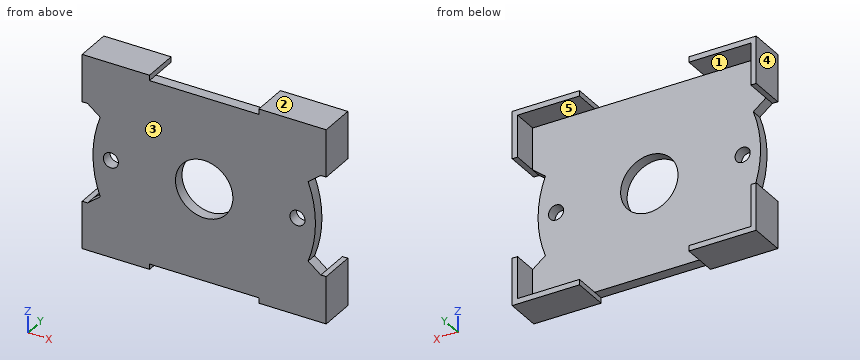
```python
from build123d import *

# Parameters (mm, degrees)
BOSS_EXTRUDE1_DEPTH   = 10
BOSS_EXTRUDE1_2_DEPTH = 10
BOSS_EXTRUDE1_3_DEPTH = 10
BOSS_EXTRUDE1_4_DEPTH = 10
SKETCH1_9_R           = 2.1
SKETCH1_9_R_2         = 22.5
SKETCH1_9_R_3         = 8
BOSS_EXTRUDE2_DEPTH   = 3


with BuildPart() as part:
    # Sketch1 → Boss-Extrude1 (new body)
    with BuildSketch(Plane(origin=(0, 0, 0), x_dir=(1, 0, 0), z_dir=(0, 1, 0))):
        Polygon((-15.231546212, -27), (-15.231546212, -25.5), (-17.628102564, -25.5), (-32.5, -25.5), (-32.5, -13.831280473), (-34, -13.831280473), (-34, -27), align=None)
    extrude(amount=BOSS_EXTRUDE1_DEPTH)



with BuildPart() as body_2:
    # Sketch1 → Boss-Extrude1 2 (new body)
    with BuildSketch(Plane(origin=(0, 0, 0), x_dir=(1, 0, 0), z_dir=(0, 1, 0))):
        Polygon((32.5, -13.831280473), (32.5, -25.5), (17.628102564, -25.5), (15.231546212, -25.5), (15.231546212, -27), (34, -27), (34, -13.831280473), align=None)
    extrude(amount=BOSS_EXTRUDE1_2_DEPTH)


with BuildPart() as body_3:
    # Sketch1 → Boss-Extrude1 3 (new body)
    with BuildSketch(Plane(origin=(0, 0, 0), x_dir=(1, 0, 0), z_dir=(0, 1, 0))):
        Polygon((32.5, 25.5), (32.5, 13.831280473), (34, 13.831280473), (34, 27), (15.231546212, 27), (15.231546212, 25.5), (17.628102564, 25.5), align=None)
    extrude(amount=BOSS_EXTRUDE1_3_DEPTH)


with BuildPart() as body_4:
    # Sketch1 → Boss-Extrude1 4 (new body)
    with BuildSketch(Plane(origin=(0, 0, 0), x_dir=(1, 0, 0), z_dir=(0, 1, 0))):
        Polygon((-17.628102564, 25.5), (-15.231546212, 25.5), (-15.231546212, 27), (-34, 27), (-34, 13.831280473), (-32.5, 13.831280473), (-32.5, 25.5), align=None)
    extrude(amount=BOSS_EXTRUDE1_4_DEPTH)


with BuildPart() as part_1:
    add(part.part)

    add(body_2.part)  # Boss-Extrude2 merges body 2

    add(body_3.part)  # Boss-Extrude2 merges body 3

    add(body_4.part)  # Boss-Extrude2 merges body 4
    # Sketch1_9 → Boss-Extrude2 (add)
    # profile 1 of 15: a face of its own
    with BuildSketch(Plane(origin=(0, 0, 0), x_dir=(1, 0, 0), z_dir=(0, 1, 0))):
        with BuildLine():
            Line((-32.5, 25.5), (-32.5, 13.831280473))
            Line((-32.5, 13.831280473), (-28.961769494, 11.055130384))
            ThreePointArc((-28.961769494, 11.055130384), (-24.388882901, 19.135892737), (-17.628102564, 25.5))
            Line((-17.628102564, 25.5), (-32.5, 25.5))
        make_face()
    # profile 2 of 15: a face of its own
    with BuildSketch(Plane(origin=(0, 0, 0), x_dir=(1, 0, 0), z_dir=(0, 1, 0))):
        with BuildLine():
            Line((-28.961769494, 11.055130384), (-21.828002387, 5.457866962))
            ThreePointArc((-21.828002387, 5.457866962), (-17.701608557, 13.888954406), (-10.494335458, 19.902736578))
            Line((-10.494335458, 19.902736578), (-17.628102564, 25.5))
            ThreePointArc((-17.628102564, 25.5), (-24.388882901, 19.135892737), (-28.961769494, 11.055130384))
        make_face()
    # profile 3 of 15: a face of its own
    with BuildSketch(Plane(origin=(0, 0, 0), x_dir=(1, 0, 0), z_dir=(0, 1, 0))):
        with BuildLine():
            Line((10.494335458, 19.902736578), (17.628102564, 25.5))
            Line((17.628102564, 25.5), (15.231546212, 25.5))
            Line((15.231546212, 25.5), (-15.231546212, 25.5))
            Line((-15.231546212, 25.5), (-17.628102564, 25.5))
            Line((-17.628102564, 25.5), (-10.494335458, 19.902736578))
            ThreePointArc((-10.494335458, 19.902736578), (0, 22.5), (10.494335458, 19.902736578))
        make_face()
    # profile 4 of 15: a face of its own
    with BuildSketch(Plane(origin=(0, 0, 0), x_dir=(1, 0, 0), z_dir=(0, 1, 0))):
        with BuildLine():
            Line((21.828002387, 5.457866962), (28.961769494, 11.055130384))
            ThreePointArc((28.961769494, 11.055130384), (24.388882901, 19.135892737), (17.628102564, 25.5))
            Line((17.628102564, 25.5), (10.494335458, 19.902736578))
            ThreePointArc((10.494335458, 19.902736578), (17.701608557, 13.888954406), (21.828002387, 5.457866962))
        make_face()
    # profile 5 of 15: a face of its own
    with BuildSketch(Plane(origin=(0, 0, 0), x_dir=(1, 0, 0), z_dir=(0, 1, 0))):
        with BuildLine():
            Line((28.961769494, 11.055130384), (32.5, 13.831280473))
            Line((32.5, 13.831280473), (32.5, 25.5))
            Line((32.5, 25.5), (17.628102564, 25.5))
            ThreePointArc((17.628102564, 25.5), (24.388882901, 19.135892737), (28.961769494, 11.055130384))
        make_face()
    # profile 6 of 15: a face of its own
    with BuildSketch(Plane(origin=(0, 0, 0), x_dir=(1, 0, 0), z_dir=(0, 1, 0))):
        with BuildLine():
            Line((21.828002387, -5.457866962), (28.961769494, -11.055130384))
            ThreePointArc((28.961769494, -11.055130384), (31, 0), (28.961769494, 11.055130384))
            Line((28.961769494, 11.055130384), (21.828002387, 5.457866962))
            ThreePointArc((21.828002387, 5.457866962), (22.331368674, 2.749540533), (22.5, 0))
            ThreePointArc((22.5, 0), (22.331368674, -2.749540533), (21.828002387, -5.457866962))
        make_face()
        with Locations(Location((26, 0, 0), (0, 0, 270))):
            Circle(SKETCH1_9_R, mode=Mode.SUBTRACT)
    # profile 7 of 15: a face of its own
    with BuildSketch(Plane(origin=(0, 0, 0), x_dir=(1, 0, 0), z_dir=(0, 1, 0))):
        with BuildLine():
            Line((-24.388882901, -19.135892737), (-17.701608557, -13.888954406))
            ThreePointArc((-17.701608557, -13.888954406), (-20.209362786, -9.890988615), (-21.828002387, -5.457866962))
            Line((-21.828002387, -5.457866962), (-28.961769494, -11.055130384))
            ThreePointArc((-28.961769494, -11.055130384), (-26.979579459, -15.267687848), (-24.388882901, -19.135892737))
        make_face()
    # profile 8 of 15: a face of its own
    with BuildSketch(Plane(origin=(0, 0, 0), x_dir=(1, 0, 0), z_dir=(0, 1, 0))):
        with BuildLine():
            Line((-28.961769494, -11.055130384), (-21.828002387, -5.457866962))
            ThreePointArc((-21.828002387, -5.457866962), (-22.5, 0), (-21.828002387, 5.457866962))
            Line((-21.828002387, 5.457866962), (-28.961769494, 11.055130384))
            ThreePointArc((-28.961769494, 11.055130384), (-31, 0), (-28.961769494, -11.055130384))
        make_face()
        with Locations(Location((-26, 0, 0), (0, 0, 270))):
            Circle(SKETCH1_9_R, mode=Mode.SUBTRACT)
    # profile 9 of 15: a face of its own
    with BuildSketch(Plane(origin=(0, 0, 0), x_dir=(1, 0, 0), z_dir=(0, 1, 0))):
        with BuildLine():
            Line((-32.5, -13.831280473), (-32.5, -25.5))
            Line((-32.5, -25.5), (-24.388882901, -19.135892737))
            ThreePointArc((-24.388882901, -19.135892737), (-26.979579459, -15.267687848), (-28.961769494, -11.055130384))
            Line((-28.961769494, -11.055130384), (-32.5, -13.831280473))
        make_face()
    # profile 10 of 15: a face of its own
    with BuildSketch(Plane(origin=(0, 0, 0), x_dir=(1, 0, 0), z_dir=(0, 1, 0))):
        with BuildLine():
            Line((-32.5, -25.5), (-17.628102564, -25.5))
            ThreePointArc((-17.628102564, -25.5), (-21.248111262, -22.572500256), (-24.388882901, -19.135892737))
            Line((-24.388882901, -19.135892737), (-32.5, -25.5))
        make_face()
    # profile 11 of 15: a face of its own
    with BuildSketch(Plane(origin=(0, 0, 0), x_dir=(1, 0, 0), z_dir=(0, 1, 0))):
        with BuildLine():
            Line((-17.628102564, -25.5), (-10.494335458, -19.902736578))
            ThreePointArc((-10.494335458, -19.902736578), (-14.415068807, -17.275873097), (-17.701608557, -13.888954406))
            Line((-17.701608557, -13.888954406), (-24.388882901, -19.135892737))
            ThreePointArc((-24.388882901, -19.135892737), (-21.248111262, -22.572500256), (-17.628102564, -25.5))
        make_face()
    # profile 12 of 15: a face of its own
    with BuildSketch(Plane(origin=(0, 0, 0), x_dir=(1, 0, 0), z_dir=(0, 1, 0))):
        with BuildLine():
            Line((15.231546212, -25.5), (17.628102564, -25.5))
            Line((17.628102564, -25.5), (10.494335458, -19.902736578))
            ThreePointArc((10.494335458, -19.902736578), (0, -22.5), (-10.494335458, -19.902736578))
            Line((-10.494335458, -19.902736578), (-17.628102564, -25.5))
            Line((-17.628102564, -25.5), (-15.231546212, -25.5))
            Line((-15.231546212, -25.5), (15.231546212, -25.5))
        make_face()
    # profile 13 of 15: a face of its own
    with BuildSketch(Plane(origin=(0, 0, 0), x_dir=(1, 0, 0), z_dir=(0, 1, 0))):
        with BuildLine():
            Line((10.494335458, -19.902736578), (17.628102564, -25.5))
            ThreePointArc((17.628102564, -25.5), (24.388882901, -19.135892737), (28.961769494, -11.055130384))
            Line((28.961769494, -11.055130384), (21.828002387, -5.457866962))
            ThreePointArc((21.828002387, -5.457866962), (17.701608557, -13.888954406), (10.494335458, -19.902736578))
        make_face()
    # profile 14 of 15: a face of its own
    with BuildSketch(Plane(origin=(0, 0, 0), x_dir=(1, 0, 0), z_dir=(0, 1, 0))):
        with BuildLine():
            Line((17.628102564, -25.5), (32.5, -25.5))
            Line((32.5, -25.5), (32.5, -13.831280473))
            Line((32.5, -13.831280473), (28.961769494, -11.055130384))
            ThreePointArc((28.961769494, -11.055130384), (24.388882901, -19.135892737), (17.628102564, -25.5))
        make_face()
    # profile 15 of 15: a face of its own
    with BuildSketch(Plane(origin=(0, 0, 0), x_dir=(1, 0, 0), z_dir=(0, 1, 0))):
        Circle(SKETCH1_9_R_2)
        with Locations(Location((0, 0, 0), (0, 0, 270))):
            Circle(SKETCH1_9_R_3, mode=Mode.SUBTRACT)
    extrude(amount=BOSS_EXTRUDE2_DEPTH)


solid = part_1.part
```
CAD build for the part. Positions are in the model's coordinates, mm. Face numbers are marked on the shaded views. A direction names the side the tool comes from. Round coordinates to 2 decimals unless told otherwise and drop trailing zeros. Loops run counter-clockwise (first coordinate to the right, second up) from the corner with the lowest first, then second, coordinate; pieces in that order, holes last. Notation, with made-up numbers: (14, -39.75) - (64, -39.75) arc R25 ccw to (64, -14.75) - close; hole circle Ø6 at (48, 60.25). An arc over 180 degrees is marked (long way). Return JSON: item names as keys, results as strings. Group by question number.
Q1. Two-plate mould, pull along X, no slides. Class the marked faces 3, 4 and 5: +X half, -X half, draft (parallel to the pull), parting line (faces both ways), or undercut.
Q2. Band-saw the part on D-D on z = -18.5. Give the cut face in (x, y).
Q3. Tool access for the marked faces 1 and 2: list every direction of +Z, -Z, +X, -X, +Y, -Y with a clear straight run to the whole face (end or side of a thin tool).
Q4. Drill centre lines: line 1 along X through (y, z) = (2.35, 0); line 2 along X through (y, z) = (6.25, -23.5); line 3 along Z through (x, y) = (-27, 8). Where is each one in solid material? Low to high. Write a range as [from, to].
Q5. Flat gauge pins, fed straight in: pin 1 Ø2.5 at (x, z) = (26, 0) entering from -Y; pin 2 Ø1 at (x, z) = (18, -15.5) entering from -Y; pin 3 Ø1 at (x, y) = (14.5, 1.5) entering from -Z; pin 4 Ø1.5 at (x, z) = (24.5, -7) entering from +Y. Where does each tip first touch, or does it go through?
Q6. Band-saw the part on B-B on x = 26. Give the cut face in (y, z), plus the area to 3 significant figures.
Q7. Band-saw the part on A-A on z = 0. Give the cut face in (x, y).
Q8. Band-saw the part on C-C on y = 4.75. Give the cut face in (x, z).
Solutions:
{
 "1": {"face 3": "draft", "face 4": "-X half", "face 5": "undercut"},
 "2": {"outline": "(-34, 0) - (34, 0) - (34, 10) - (32.5, 10) - (32.5, 3) - (-32.5, 3) - (-32.5, 10) - (-34, 10) - close"},
 "3": {"face 1": "+Y", "face 2": "+Z, +X, -X, +Y, -Y"},
 "4": {"line 1": "x = [-31, -28.1], [-23.9, -8], [8, 23.9], [28.1, 31]", "line 2": "x = [-34, -32.5], [32.5, 34]", "line 3": "z = [-27, -25.5], [25.5, 27]"},
 "5": {"pin 1": "passes through", "pin 2": "stops at y = 0", "pin 3": "stops at z = -25.5", "pin 4": "stops at y = 3"},
 "6": {"outline": "(0, -27) - (10, -27) - (10, -25.5) - (3, -25.5) - (3, -2.1) - (0, -2.1) - close; (0, 2.1) - (3, 2.1) - (3, 25.5) - (10, 25.5) - (10, 27) - (0, 27) - close", "area": "170 mm^2"},
 "7": {"outline": "(-31, 0) - (-28.1, 0) - (-28.1, 3) - (-31, 3) - close; (-23.9, 0) - (-8, 0) - (-8, 3) - (-23.9, 3) - close; (8, 0) - (23.9, 0) - (23.9, 3) - (8, 3) - close; (28.1, 0) - (31, 0) - (31, 3) - (28.1, 3) - close"},
 "8": {"outline": "(-34, -27) - (-15.23, -27) - (-15.23, -25.5) - (-32.5, -25.5) - (-32.5, -13.83) - (-34, -13.83) - close; (-34, 13.83) - (-32.5, 13.83) - (-32.5, 25.5) - (-15.23, 25.5) - (-15.23, 27) - (-34, 27) - close; (15.23, -27) - (34, -27) - (34, -13.83) - (32.5, -13.83) - (32.5, -25.5) - (15.23, -25.5) - close; (15.23, 25.5) - (32.5, 25.5) - (32.5, 13.83) - (34, 13.83) - (34, 27) - (15.23, 27) - close"}
}
